The listing builds one solid part. Answer for the finished solid, in the listing's coordinates (mm). A direction names the side the tool comes from. Round coordinates to 2 decimals unless told otherwise and drop trailing zeros. Write each loop counter-clockwise with the first axis right and the second up, starting at its lowest first coordinate (ties: lowest second). Pieces come first, ordered by that corner, then holes. Notation, with made-up numbers: (-6, 44) - (46, 44) arc R22 ccw to (46, 72) - close; hole circle Ø2 at (49, 70). An arc over 180 degrees is marked (long way). Return JSON: item names as keys, results as strings. Group by question number.
from build123d import *

# Parameters (mm, degrees)
SALIENTE_EXTRUIR3_DEPTH    = 5
CORTAR_EXTRUIR2_DEPTH      = 11.978246956
CORTAR_EXTRUIR2_DEPTH_BACK = 11.978246956
CROQUIS5_R                 = 0.625
CROQUIS7_W                 = 24
CROQUIS7_H                 = 24
SALIENTE_EXTRUIR5_DEPTH    = 3.5


with BuildPart() as part:
    # Croquis1 → Saliente-Extruir3 (new body)
    with BuildSketch(Plane.XY):
        with BuildLine():
            ThreePointArc((5.390964663, 2), (-0.132231752, 5.748479344), (-5.477225575, 1.75))
            Line((-5.477225575, 1.75), (-3.596873642, 1.75))
            ThreePointArc((-3.596873642, 1.75), (0.897915762, 3.897915762), (4, 0))
            ThreePointArc((4, 0), (0.897915762, -3.897915762), (-3.596873642, -1.75))
            Line((-3.596873642, -1.75), (-5.477225575, -1.75))
            ThreePointArc((-5.477225575, -1.75), (-0.132231752, -5.748479344), (5.390964663, -2))
            Line((5.390964663, -2), (4.749257399, -2))
            Line((4.749257399, -2), (4.749257399, 2))
            Line((4.749257399, 2), (5.390964663, 2))
        make_face()
        with BuildLine():
            Line((-5.748043145, -0.15), (-7.903126358, -0.15))
            Line((-7.903126358, -0.15), (-7.903126358, -1.75))
            Line((-7.903126358, -1.75), (-5.477225575, -1.75))
            ThreePointArc((-5.477225575, -1.75), (-5.66936191, -0.959601761), (-5.748043145, -0.15))
        make_face()
        with BuildLine():
            Line((-5.477225575, 1.75), (-7.903126358, 1.75))
            Line((-7.903126358, 1.75), (-7.903126358, 0.15))
            Line((-7.903126358, 0.15), (-5.748043145, 0.15))
            ThreePointArc((-5.748043145, 0.15), (-5.66936191, 0.959601761), (-5.477225575, 1.75))
        make_face()
        with BuildLine():
            Line((-3.596873642, 1.75), (-5.477225575, 1.75))
            ThreePointArc((-5.477225575, 1.75), (-5.66936191, 0.959601761), (-5.748043145, 0.15))
            Line((-5.748043145, 0.15), (-3.997186511, 0.15))
            ThreePointArc((-3.997186511, 0.15), (-3.880391398, 0.970856631), (-3.596873642, 1.75))
        make_face()
        with BuildLine():
            Line((-3.997186511, -0.15), (-5.748043145, -0.15))
            ThreePointArc((-5.748043145, -0.15), (-5.66936191, -0.959601761), (-5.477225575, -1.75))
            Line((-5.477225575, -1.75), (-3.596873642, -1.75))
            ThreePointArc((-3.596873642, -1.75), (-3.880391398, -0.970856631), (-3.997186511, -0.15))
        make_face()
        with BuildLine():
            Line((6.750742601, 2), (5.390964663, 2))
            ThreePointArc((5.390964663, 2), (5.659529433, 1.015985528), (5.75, 0))
            ThreePointArc((5.75, 0), (5.659529433, -1.015985528), (5.390964663, -2))
            Line((5.390964663, -2), (6.750742601, -2))
            Line((6.750742601, -2), (6.750742601, 2))
        make_face()
        with BuildLine():
            ThreePointArc((5.75, 0), (5.659529433, 1.015985528), (5.390964663, 2))
            Line((5.390964663, 2), (4.749257399, 2))
            Line((4.749257399, 2), (4.749257399, -2))
            Line((4.749257399, -2), (5.390964663, -2))
            ThreePointArc((5.390964663, -2), (5.659529433, -1.015985528), (5.75, 0))
        make_face()
    extrude(amount=SALIENTE_EXTRUIR3_DEPTH)

    # Croquis5 → Cortar-Extruir2 (cut, two sides: drawn at the far end of the back side and taken through both)
    with BuildSketch(Plane(origin=(0, 0, 0), x_dir=(1, 0, 0), z_dir=(0, 1, 0)).offset(-CORTAR_EXTRUIR2_DEPTH_BACK)):
        with Locations(Location((-6.690175966, -2.5, 0), (0, 0, 270))):
            Circle(CROQUIS5_R)
    extrude(amount=CORTAR_EXTRUIR2_DEPTH + CORTAR_EXTRUIR2_DEPTH_BACK, mode=Mode.SUBTRACT)

    # Croquis7 → Saliente-Extruir5 (add)
    with BuildSketch(Plane(origin=(6.750742601, 0, 0), x_dir=(0, 0, -1), z_dir=(1, 0, 0))):
        with Locations((-2.5, 0)):
            Rectangle(CROQUIS7_W, CROQUIS7_H)
    extrude(amount=SALIENTE_EXTRUIR5_DEPTH)


solid = part.part
(1) Find section B-B (x = -2.25). Write down the section's boundary in (y, z), plus the area to 3 significant figures.
(2) Find section A-A (z = 2.5). Write down the section's boundary in (x, y).
(3) Consider line 1 (X direction, y = -1.2, z = 2.5); line 2 (X direction, y = -0.95, z = 2.5); line 3 (X direction, y = 0, z = -7.25). Determine where each line is inside the solid, lowest interval first.
(4) Find section C-C (y = -10). Write down the section's boundary in (x, z), plus the area to 3 significant figures.
(5) For faces 1 (the flat face through (-6, 1.75, 2)), 2 (the flat face through (-6, 0.15, 2)), 3 (the flat face through (6, -2, 2)), 4 (the flat face through (-3.94, 1.36, 5)), 5 (the flat face through (-3.94, 1.36, 0)), determine the directions among +Z, -Z, +X, -X, +Y, -Y from which every point of the face is accessible in a straight line to the end or side of a thin tool.
(6) Determine the mould class of faces 6 (the flat face through (6, 2, 2)), 7 (the flat face through (10.251, 0, 3)), 8 (the flat face through (-7.903, 1, 2)), 9 (the flat face through (8, 0, -9.5)) for opening direction X: +X half, -X half, draft (parallel to the pull), parting line (faces both ways), or undercut.
(7) Flat-ended cylindrical pins translate along their axes: pin 1 (1.4 mm diameter, centred on x = -6.69, z = 2.5, fed in from +Y); pin 2 (1.1 mm diameter, centred on x = 6, z = 3, fed in from +Y); pin 3 (1.5 mm diameter, centred on x = 3, y = 2, fed in from -Z); pin 4 (12 mm diameter, centred on y = 2, z = 4, fed in from -X). Find the tip coordinate at first contact, or state that the pin passes through.
(8) Find section D-D (x = 6). Write down the section's boundary in (y, z), plus the area to 3 significant figures.
Check sheet entries:
{
 "1": {"outline": "(-5.29, 0) - (-3.31, 0) - (-3.31, 5) - (-5.29, 5) - close; (3.31, 0) - (5.29, 0) - (5.29, 5) - (3.31, 5) - close", "area": "19.8 mm^2"},
 "2": {"outline": "(-7.9, -1.75) - (-7.32, -1.75) - (-7.32, -0.15) - (-7.9, -0.15) - close; (-7.9, 0.15) - (-7.32, 0.15) - (-7.32, 1.75) - (-7.9, 1.75) - close; (-6.07, -1.75) - (-5.48, -1.75) arc R5.75 ccw to (5.39, -2) - (6.75, -2) - (6.75, -12) - (10.25, -12) - (10.25, 12) - (6.75, 12) - (6.75, 2) - (5.39, 2) arc R5.75 ccw to (-5.48, 1.75) - (-6.07, 1.75) - (-6.07, 0.15) - (-4, 0.15) arc R4 cw (long way) to (-4, -0.15) - (-6.07, -0.15) - close"},
 "3": {"line 1": "x = -7.9 to -7.32, -6.07 to -3.82, 3.82 to 10.25", "line 2": "x = -7.9 to -7.32, -6.07 to -3.89, 3.89 to 10.25", "line 3": "x = 6.75 to 10.25"},
 "4": {"outline": "(6.75, -9.5) - (10.25, -9.5) - (10.25, 14.5) - (6.75, 14.5) - close", "area": "84.0 mm^2"},
 "5": {"face 1": "+Z, -Z, -X, +Y", "face 2": "+Z, -Z, -X", "face 3": "+Z, -Z, -Y", "face 4": "+Z, -X, +Y, -Y", "face 5": "-Z, -X, +Y, -Y"},
 "6": {"face 6": "undercut", "face 7": "+X half", "face 8": "-X half", "face 9": "draft"},
 "7": {"pin 1": "stops at y = 1.75", "pin 2": "stops at y = 2", "pin 3": "stops at z = 0", "pin 4": "stops at x = -7.9"},
 "8": {"outline": "(-2, 0) - (2, 0) - (2, 5) - (-2, 5) - close", "area": "20.0 mm^2"}
}
